Autodesk Inventor part; units mm, degrees
ref_plane "YZ Plane" through (0, 0, 0) normal (1, 0, 0) x (0, 1, 0)
ref_plane "XZ Plane" through (0, 0, 0) normal (0, 1, 0) x (-1, 0, 0)
ref_plane "XY Plane" through (0, 0, 0) normal (0, 0, 1) x (1, 0, 0)
sketch "Sketch1" plane through (0, 0, 0) normal (0, 1, 0) x (-1, 0, 0)
  line L0 (50.1781, 160.1313) -> (-129.8219, 160.1313)
  line L1 (-129.8219, 160.1313) -> (-129.8219, -99.8687)
  line L2 (-129.8219, -99.8687) -> (50.1781, -99.8687)
  line L3 (50.1781, -99.8687) -> (50.1781, 160.1313)
  point P0 (0, 0)
  dimension "d0" = 260
  dimension "d1" = 180
extrude "Extrusion1" add sketch "Sketch1" along normal blind 5
sketch "Sketch2" plane through (0, 0, 0) normal (0, -1, 0) x (1, 0, 0)
  line L0 (129.8219, 160.1313) -> (129.8219, -99.8687)
  line L1 (-50.1781, -99.8687) -> (-50.1781, 160.1313)
  line L2 (129.8219, 160.1313) -> (-50.1781, 160.1313)
  line L3 (-50.1781, 160.1313) -> (-50.1781, 155.1313)
  line L4 (-50.1781, 155.1313) -> (129.8219, 155.1313)
  line L5 (129.8219, 155.1313) -> (129.8219, 160.1313)
  line L6 (129.8219, -99.8687) -> (-50.1781, -99.8687)
  line L7 (-50.1781, -99.8687) -> (-50.1781, -94.8687)
  line L8 (-50.1781, -94.8687) -> (129.8219, -94.8687)
  line L9 (129.8219, -94.8687) -> (129.8219, -99.8687)
  point P0 (0, 0)
  point P1 (129.8219, 155.1313)
  dimension "d4" = 5
  dimension "d5" = 5
extrude "Extrusion2" add sketch "Sketch2" along normal blind 7 contours L0 L4 L1 L2 | L0 L6 L1 L8
sketch "Sketch3" plane through (0, 5, 0) normal (0, 1, 0) x (1, 0, 0)
  line L0 (109.8219, 29.8687) -> (-30.1781, 29.8687)
  line L1 (-30.1781, 29.8687) -> (-30.1781, -90.1313)
  line L2 (-30.1781, -90.1313) -> (109.8219, -90.1313)
  line L3 (109.8219, -90.1313) -> (109.8219, 29.8687)
  line L4 (129.8219, -160.1313) -> (129.8219, 99.8687)
  line L5 (-50.1781, 99.8687) -> (-50.1781, -160.1313)
  line L6 (-50.1781, -160.1313) -> (129.8219, -160.1313)
  line L7 (129.8219, 99.8687) -> (-50.1781, 99.8687)
  point P0 (0, 0)
  dimension "d8" = 20
  dimension "d9" = 20
  dimension "d10" = 70
  dimension "d11" = 70
extrude "Extrusion3" cut sketch "Sketch3" against normal through all contours L3 L2 L1 L0
properties part number "machine_platform"
Check sheet for the modelled part. Datum: model origin and axes. Units: mm. A direction names the side the tool comes from. Coordinates: 2 decimals unless noted, no trailing zeros. Loops run counter-clockwise (first coordinate to the right, second up) from the corner with the lowest first, then second, coordinate; pieces in that order, holes last. Notation, with made-up numbers: (48, -19.5) -> (89, -19.5) arc R25 cw to (89, 8.5) -> close; hole circle Ø9 at (51.5, 75.5). An arc over 180 degrees is marked (long way). Write item = value, one per line. Start each with the question number.
1. Section check A-A on y = 2.5. Record the cut outline in (x, z).
2. Tool access check on faces 4 (the flat face through (39, 3, 90.131)), 5 (the flat face through (-50.178, 3, 28)), 6 (the flat face through (39, -3, 155.131)). Record the directions out of +Z, -Z, +X, -X, +Y, -Y that give a thin tool (end or side, any length) a straight path to the whole face; none if there is none.
3. Section check C-C on x = 59. Record the cut outline in (y, z).
4. Material ranges on line 1 (X direction, y = 4, z = 40.5); line 2 (Z direction, x = 66, y = 2.75); line 3 (Z direction, x = 107.5, y = -1.25), recorded low to high.
5. Draft check along Z on faces 1 (the flat face through (-30.178, 3, 29)), 2 (the flat face through (39, -1, 160.131)), 3 (the flat face through (41, -1, -99.869)). Enter one of: released by +Z, released by -Z, zero draft, split by the parting line, or undercut.
6. Section check B-B on z = 84. Record the cut outline in (x, y).
Responses:
q1.outline = (-50.18, -99.87) -> (129.82, -99.87) -> (129.82, 160.13) -> (-50.18, 160.13) -> close; hole (-30.18, -29.87) -> (109.82, -29.87) -> (109.82, 90.13) -> (-30.18, 90.13) -> close
q2.face_4 = +Y, -Y
q2.face_5 = +Z, -Z, -X, +Y, -Y
q2.face_6 = +X, -X, -Y
q3.outline = (-7, -99.87) -> (5, -99.87) -> (5, -29.87) -> (0, -29.87) -> (0, -94.87) -> (-7, -94.87) -> close; (-7, 155.13) -> (0, 155.13) -> (0, 90.13) -> (5, 90.13) -> (5, 160.13) -> (-7, 160.13) -> close
q4.line_1 = -50.18 to -30.18, 109.82 to 129.82
q4.line_2 = -99.87 to -29.87, 90.13 to 160.13
q4.line_3 = -99.87 to -94.87, 155.13 to 160.13
q5.face_1 = undercut
q5.face_2 = released by +Z
q5.face_3 = released by -Z
q6.outline = (-50.18, 0) -> (-30.18, 0) -> (-30.18, 5) -> (-50.18, 5) -> close; (109.82, 0) -> (129.82, 0) -> (129.82, 5) -> (109.82, 5) -> close
